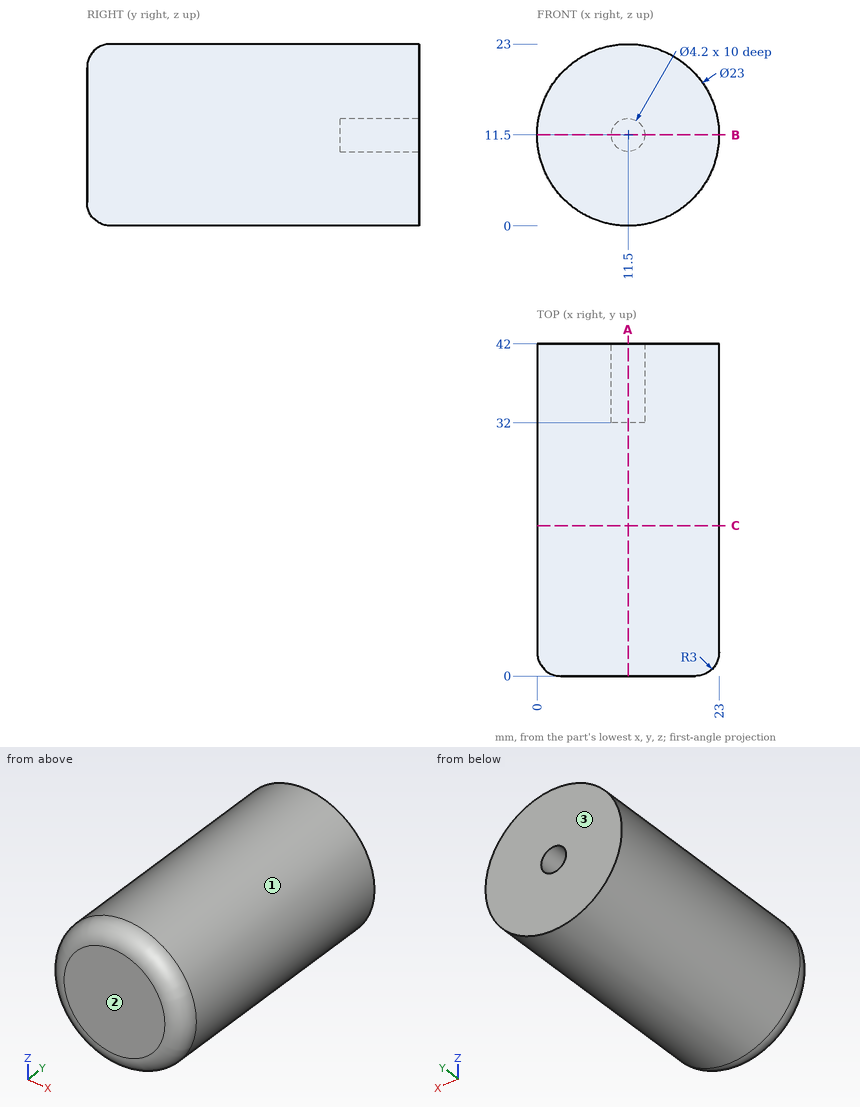
Source: three-view drawing plus pictorial views. Frame: mm from the lowest corner of the part. Round coordinates to 2 decimals unless told otherwise and drop trailing zeros. Loops run counter-clockwise (first coordinate to the right, second up) from the corner with the lowest first, then second, coordinate; pieces in that order, holes last. Notation, with made-up numbers: M -33.75,27 L 9.25,27 A26 ccw 9.25,43 Z; hole C 84.5,25 d7. An arc over 180 degrees is marked long. Answer as CSV lines item,"result". Start each with the question number.
(1) Section A-A, the plane x = 11.5. Output: boundary loops of the cut face in (y, z), plus the area to 3 significant figures.
(2) Line query: line 1 (X direction, y = 40, z = 11.5); line 2 (X direction, y = 25.5, z = 11.25). Output: solid intervals per line, ascending. Write a range as [from, to].
(3) Draft query along Y for the marked faces 1, 2 and 3. Return one class per face: released by +Y, released by -Y, zero draft, split by the parting line, or undercut.
(4) Section B-B, the plane z = 11.5. Output: boundary loops of the cut face in (x, y), plus the area to 3 significant figures.
(5) Section C-C, the plane y = 19. Output: boundary loops of the cut face in (x, z), plus the area to 3 significant figures.
(6) First-contact query: pin 1 (8 mm diameter, centred on x = 17.5, y = 30, fed in from +Z); pin 2 (10 mm diameter, centred on x = 20, y = 24.5, fed in from -Z). Flat tips, straight axial feed; report the tip coordinate or a pass-through.
Values found:
1,outline,"M 0,3 A3 ccw 3,0 L 42,0 L 42,9.4 L 32,9.4 L 32,13.6 L 42,13.6 L 42,23 L 3,23 A3 ccw 0,20 Z"
1,area,"920 mm²"
2,line 1,"x = [0, 9.4], [13.6, 23]"
2,line 2,"x = [0, 23]"
3,face 1,"zero draft"
3,face 2,"released by -Y"
3,face 3,"released by +Y"
4,outline,"M 0,3 A3 ccw 3,0 L 20,0 A3 ccw 23,3 L 23,42 L 13.6,42 L 13.6,32 L 9.4,32 L 9.4,42 L 0,42 Z"
4,area,"920 mm²"
5,outline,"C 11.5,11.5 d23"
5,area,"415 mm²"
6,pin 1,"stops at z = 22.82"
6,pin 2,"stops at z = 0.55"
